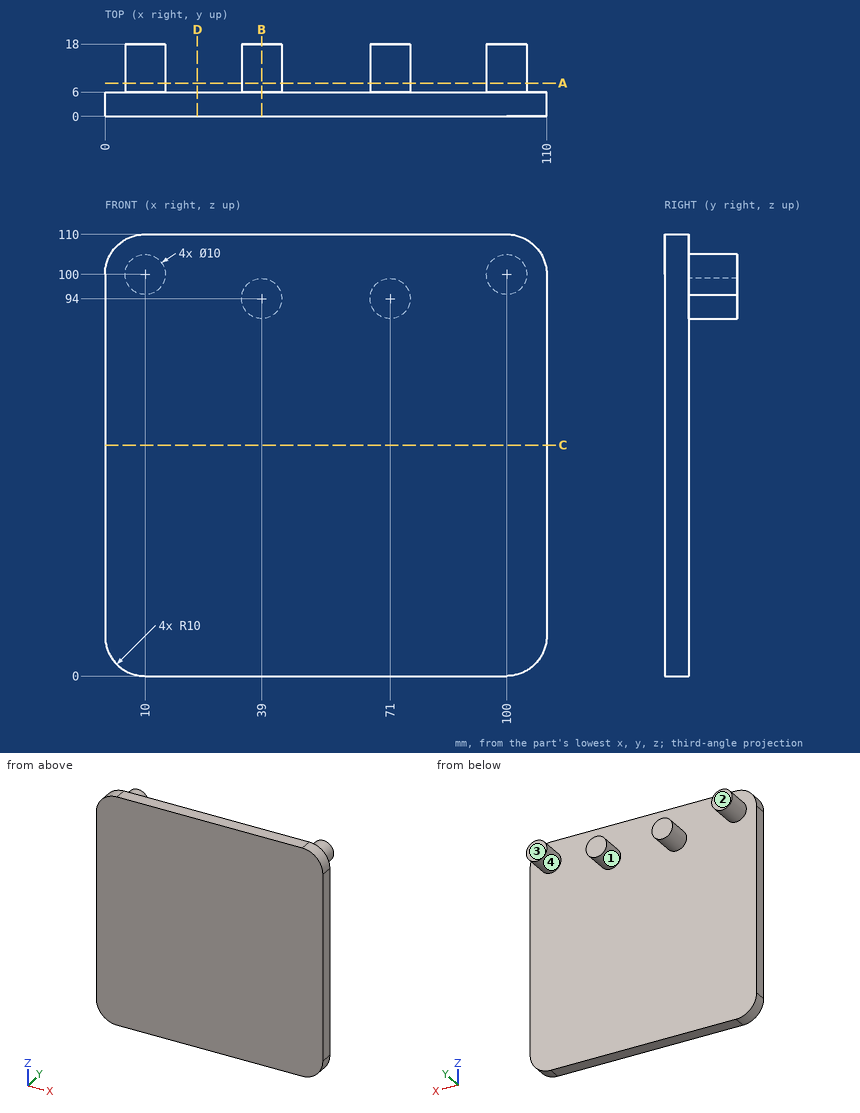
Input: dimensioned drawing with shaded views. Units: mm. Origin: part minimum x, y, z. A direction names the side the tool comes from. Coordinates: 2 decimals unless noted, no trailing zeros. Order: outer loops, then holes, each group sorted by start corner. A loop starts at its lowest first (then second) coordinate and runs counter-clockwise, first axis right, second up.
(1) Section query B-B (x = 39). Return the cut outline in (y, z), plus the area to 3 significant figures.
(2) Material intervals for probe 1 along Y at (x, z) = (78, 82); probe 2 along X at (y, z) = (10.5, 90.5); probe 3 along Z at (x, y) = (36.5, 9.25), sorted ascending.
(3) Draft query along X for the marked faces 3 and 4. Return one class per face: pulls with the +X half, pulls with the -X half, needs draft (parallel to the pull), parting line crosses it, or undercut.
(4) Section query A-A (y = 8.25). Return the cut outline in (x, z).
(5) Section query C-C (z = 57.5). Return the cut outline in (x, y), plus the area to 3 significant figures.
(6) Access query for the marked faces 1 and 2. Directions: +Z, -Z, +X, -X, +Y, -Y. A direction counts if a zero-diameter tool reaches every point of the face in a straight line with its end or side. Return the directions, or none.
(7) Section query D-D (x = 23). Return the cut outline in (y, z), plus the area to 3 significant figures.
(8) First-contact query: pin 1 (3 mm diameter, centred on x = 35.5, y = 12.5, fed in from -Z); pin 2 (8 mm diameter, centred on y = 5, z = 18, fed in from -X); pin 3 (8 mm diameter, centred on x = 36.5, y = 15.5, fed in from +Z); pin 4 (6 mm diameter, centred on x = 43.5, y = 12, fed in from +Z). Flat tips, straight axial feed; report the tip coordinate or a pass-through.
Solution:
1. outline: (0, 0) - (6, 0) - (6, 89) - (18, 89) - (18, 99) - (6, 99) - (6, 110) - (0, 110) - close
1. area: 780 mm2
2. probe 1: y = 0 to 6
2. probe 2: x = 35.43 to 42.57, 67.43 to 74.57
2. probe 3: z = 89.67 to 98.33
3. face 3: needs draft
3. face 4: undercut
4. outline: circle Ø10 at (10, 100); circle Ø10 at (39, 94); circle Ø10 at (71, 94); circle Ø10 at (100, 100)
5. outline: (0, 0) - (110, 0) - (110, 6) - (0, 6) - close
5. area: 660 mm2
6. face 1: +Y
6. face 2: +Z, -Z, +X, -X, +Y
7. outline: (0, 0) - (6, 0) - (6, 110) - (0, 110) - close
7. area: 660 mm2
8. pin 1: stops at z = 89.42
8. pin 2: stops at x = 0
8. pin 3: stops at z = 99
8. pin 4: stops at z = 98.77
